from build123d import *

# Parameters (mm, degrees)
F1_DEPTH = 25.4
F2_DEPTH = 25.4


with BuildPart() as f1:
    # F0 (on Front) → F1 (new body)
    with BuildSketch(Plane.XZ):
        Polygon((152.4, -23.147755), (152.4, 23.147755), (-152.4, 23.147755), (-152.4, -23.147755), (-90.959854, -23.147755), (-52.855045, -23.147755), (52.855045, -23.147755), (90.959854, -23.147755), align=None)
    extrude(amount=F1_DEPTH)

    # F0 (on Front) → F2 (join)
    with BuildSketch(Plane.XZ):
        Polygon((110.626854, -91.442767), (90.959854, -23.147755), (52.855045, -23.147755), (72.522044, -91.442767), align=None)
        Polygon((-52.855045, -23.147755), (-90.959854, -23.147755), (-110.626854, -91.442767), (-72.522044, -91.442767), align=None)
    extrude(amount=F2_DEPTH)


solid = f1.part
Design review of the part built by this model. Coordinates are the model's own, in mm. A direction names the side the tool comes from. Coordinates: 2 decimals unless noted, no trailing zeros. Loops run counter-clockwise (first coordinate to the right, second up) from the corner with the lowest first, then second, coordinate; pieces in that order, holes last.
Item 1: Add section B-B (z = -70.5). Write out the cut boundary in (x, y).
Completed:
outline: (-104.6, -25.4) - (-66.49, -25.4) - (-66.49, 0) - (-104.6, 0) - close; (66.49, -25.4) - (104.6, -25.4) - (104.6, 0) - (66.49, 0) - close
Item 2: Wall thickness on L1, parallel to Z at x = -7.5, y = -18; L2, parallel to X at y = -23.5, z = -57; L3, parallel to X at y = -3.25, z = -42: over which ranges is each line inside the solid? List them lowest first.
Completed:
L1: z = -23.15 to 23.15
L2: x = -100.71 to -62.6, 62.6 to 100.71
L3: x = -96.39 to -58.28, 58.28 to 96.39
Item 3: Add section C-C (x = -122). Write out the cut boundary in (y, z), and give its area (3 significant figures).
Completed:
outline: (-25.4, -23.15) - (0, -23.15) - (0, 23.15) - (-25.4, 23.15) - close
area: 1,180 mm2
Item 4: Add section A-A (y = -8.75). Write out the cut boundary in (x, z), and give its area (3 significant figures).
Completed:
outline: (-152.4, -23.15) - (-90.96, -23.15) - (-110.63, -91.44) - (-72.52, -91.44) - (-52.86, -23.15) - (52.86, -23.15) - (72.52, -91.44) - (110.63, -91.44) - (90.96, -23.15) - (152.4, -23.15) - (152.4, 23.15) - (-152.4, 23.15) - close
area: 19,300 mm2
Item 5: Draft analysis for pull direction Z (two halves, no side actions). For faces 6 (the flat face through (100.93, -12.52, -57.77)), 7 (the flat face through (-1, -13, -23.148)), 8 (the flat face through (-122, -13, -23.148)), 9 (the flat face through (2, -13, 23.148)), state which applies: pulls with the +Z half, pulls with the -Z half, needs draft (parallel to the pull), parting line crosses it, or undercut.
Completed:
face 6: undercut
face 7: pulls with the -Z half
face 8: undercut
face 9: pulls with the +Z half
Item 6: Add section D-D (x = -57.5). Write out the cut boundary in (y, z), and give its area (3 significant figures).
Completed:
outline: (-25.4, -39.28) - (0, -39.28) - (0, 23.15) - (-25.4, 23.15) - close
area: 1,590 mm2
Item 7: For faces 1 (the flat face through (62.55, -12.52, -56.82)), 2 (the flat face through (-100.656, -12.522, -56.817)), 3 (the flat face through (121, -13, -23.148)), 4 (the flat face through (-2, -25.4, -21)), 5 (the flat face through (91, -13, -91.443)), list the 3-axis set-ups (+Z, -Z, +X, -X, +Y, -Y) from which the entire face can be reached by the end or side of a thin tool; tool diameter is ignored.
Completed:
face 1: -Z, +Y, -Y
face 2: -X, +Y, -Y
face 3: +X, +Y, -Y
face 4: +Z, -Z, +X, -X, -Y
face 5: -Z, +X, -X, +Y, -Y
Item 8: Clearance check with flat-ended pins moving along their axes: pin 1 (3 mm diameter, centred on y = -5, z = -78, fed in from -X); pin 2 (12.5 mm diameter, centred on x = 10.5, y = -11.5, fed in from -Z); pin 3 (3 mm diameter, centred on y = -16.5, z = -30.5, fed in from -X). State where each tip first meets the part, or that it passes through.
Completed:
pin 1: stops at x = -107.19
pin 2: stops at z = -23.15
pin 3: stops at x = -93.51
